Geometry check sheet. Reference: drawing and pictorial views, mm from the part's lowest x, y, z. A direction names the side the tool comes from. Round coordinates to 2 decimals unless told otherwise and drop trailing zeros. Order: outer loops, then holes, each group sorted by start corner. A loop starts at its lowest first (then second) coordinate and runs counter-clockwise, first axis right, second up.
(1) Sectioned sample at C-C, the plane z = 51.5. Enter the section's corners in (x, y).
(2) Depth check by flat-ended pin: pin 1 (8 mm diameter, centred on y = 6.5, z = 49.5, fed in from -X); pin 2 (2 mm diameter, centred on x = 11.5, z = 18, fed in from +Y); pin 3 (2 mm diameter, centred on x = 31.5, y = 33.5, fed in from -Z). Enter the tip coordinate at first touch or a pass-through.
(3) Sectioned sample at A-A, the plane x = 33.5. Enter the section's corners in (y, z), and give its area (3 significant figures).
(4) Tool access check on the marked faces 1, 2 and 3. Record the directions out of +Z, -Z, +X, -X, +Y, -Y that give a thin tool (end or side, any length) a straight path to the whole face; none if there is none.
(5) Thickness scan on probe 1 along X at (y, z) = (9, 33); probe 2 along Z at (x, y) = (3, 15.5). Record the ranges inside material, lowest first.
(6) Sectioned sample at B-B, the plane y = 23. Enter the section's corners in (x, z), and give its area (3 significant figures).
(7) Sectioned sample at D-D, the plane y = 14. Enter the section's corners in (x, z).
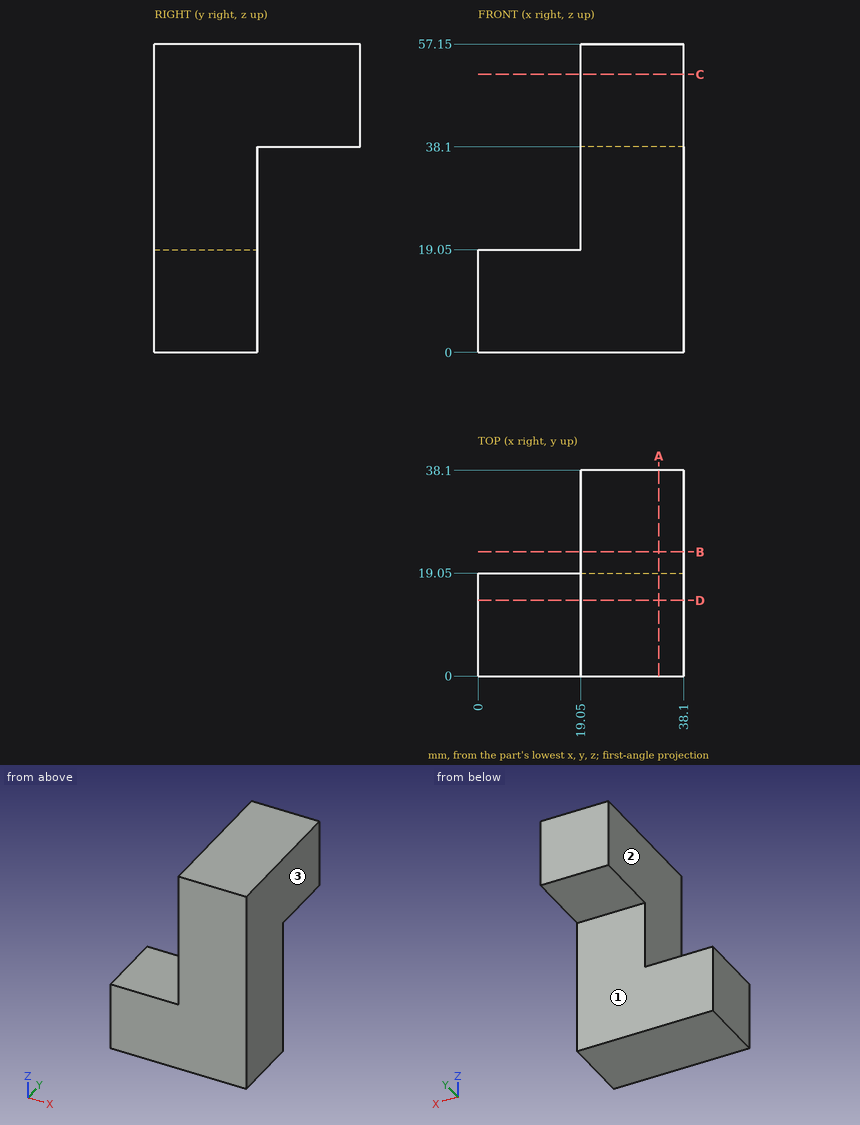
Derived:
1. outline: (19.05, 0) - (38.1, 0) - (38.1, 38.1) - (19.05, 38.1) - close
2. pin 1: stops at x = 19.05
2. pin 2: stops at y = 19.05
2. pin 3: stops at z = 38.1
3. outline: (0, 0) - (19.05, 0) - (19.05, 38.1) - (38.1, 38.1) - (38.1, 57.15) - (0, 57.15) - close
3. area: 1,450 mm2
4. face 1: -Z, +X, -X, +Y
4. face 2: +Z, -X, +Y, -Y
4. face 3: +Z, -Z, +X, +Y, -Y
5. probe 1: x = 19.05 to 38.1
5. probe 2: z = 0 to 19.05
6. outline: (19.05, 38.1) - (38.1, 38.1) - (38.1, 57.15) - (19.05, 57.15) - close
6. area: 363 mm2
7. outline: (0, 0) - (38.1, 0) - (38.1, 57.15) - (19.05, 57.15) - (19.05, 19.05) - (0, 19.05) - close
